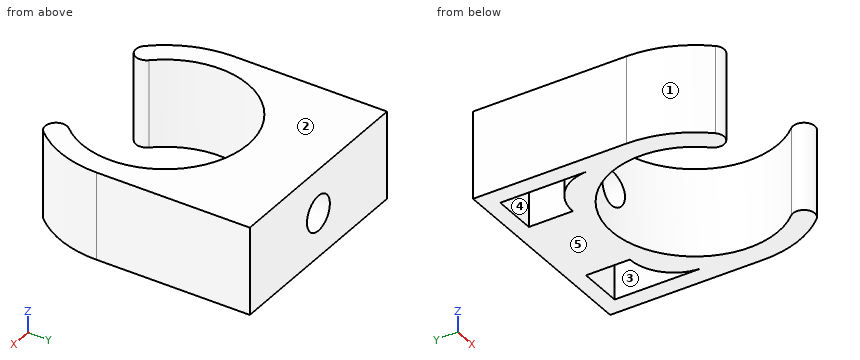
from build123d import *

# Parameters (mm, degrees)
BOSS_EXTRUDE2_DEPTH = 5
SKETCH5_R           = 2
CUT_EXTRUDE1_DEPTH  = 9
CUT_EXTRUDE2_DEPTH  = 8


with BuildPart() as part:
    # Sketch3 → Boss-Extrude2 (new, symmetric)
    with BuildSketch(Plane.XY):
        with BuildLine():
            Line((-12, -4.5), (-12, 13))
            Line((-12, 13), (12, 13))
            Line((12, 13), (12, -4.5))
            ThreePointArc((12, -4.5), (11.187544084, -8.840375258), (8.860190437, -12.593023256))
            ThreePointArc((8.860190437, -12.593023256), (7.094230677, -12.672936504), (7.014317429, -10.906976744))
            ThreePointArc((7.014317429, -10.906976744), (0, 5), (-7.014317429, -10.906976744))
            ThreePointArc((-7.014317429, -10.906976744), (-7.094230677, -12.672936504), (-8.860190437, -12.593023256))
            ThreePointArc((-8.860190437, -12.593023256), (-11.187544084, -8.840375258), (-12, -4.5))
        make_face()
    extrude(amount=BOSS_EXTRUDE2_DEPTH, both=True)

    # Sketch5 → Cut-Extrude1 (cut)
    with BuildSketch(Plane(origin=(0, 13, 0), x_dir=(1, 0, 0), z_dir=(0, 1, 0))):
        with Locations(Location((0, 0, 0), (0, 0, 270))):
            Circle(SKETCH5_R)
    extrude(amount=-CUT_EXTRUDE1_DEPTH, mode=Mode.SUBTRACT)

    # Sketch7 → Cut-Extrude2 (cut)
    with BuildSketch(Plane(origin=(0, 0, -5), x_dir=(-1, 0, 0), z_dir=(0, 0, -1))):
        with BuildLine():
            Line((10, 11.190527755), (10, 1.190527755))
            ThreePointArc((10, 1.190527755), (8.535533906, 4.726061661), (5, 6.190527755))
            Line((5, 6.190527755), (5, 11.190527755))
            Line((5, 11.190527755), (10, 11.190527755))
        make_face()
        with BuildLine():
            Line((-10, 11.190527755), (-10, 1.190527755))
            ThreePointArc((-10, 1.190527755), (-8.535533906, 4.726061661), (-5, 6.190527755))
            Line((-5, 6.190527755), (-5, 11.190527755))
            Line((-5, 11.190527755), (-10, 11.190527755))
        make_face()
    extrude(amount=-CUT_EXTRUDE2_DEPTH, mode=Mode.SUBTRACT)


solid = part.part
The model under review builds one solid part; all positions refer to its coordinate system, in mm. Face numbers are marked on the shaded views. A direction names the side the tool comes from. Coordinates: 2 decimals unless noted, no trailing zeros. Write each loop counter-clockwise with the first axis right and the second up, starting at its lowest first coordinate (ties: lowest second). Pieces come first, ordered by that corner, then holes. Notation, with made-up numbers: M 65.5,7 L 88.5,7 A27 cw 88.5,34 Z; hole C 42,72.25 d11. An arc over 180 degrees is marked long. Put each result on its own line as item: value.
1) For the marked faces 4 and 5, list the 3-axis set-ups (+Z, -Z, +X, -X, +Y, -Y) from which the entire face can be reached by the end or side of a thin tool; tool diameter is ignored.
Computed:
face 4: -Z
face 5: -Z, +X, -X, +Y, -Y
2) Add section A-A on z = 0. Give the boundary of the cut face in (x, y).
Computed:
outline: M -12,-4.5 A12 ccw -8.86,-12.59 A1.25 ccw -7.01,-10.91 A9.5 cw -2,4.79 L -2,13 L -12,13 Z; M 2,4.79 A9.5 cw 7.01,-10.91 A1.25 ccw 8.86,-12.59 A12 ccw 12,-4.5 L 12,13 L 2,13 Z; hole M -10,1.19 A5 cw -5,6.19 L -5,11.19 L -10,11.19 Z; hole M 5,6.19 A5 cw 10,1.19 L 10,11.19 L 5,11.19 Z
3) Add section D-D on y = 8. Give the boundary of the cut face in (x, z), then the cut area to 3 significant figures.
Computed:
outline: M -12,-5 L -10,-5 L -10,3 L -5,3 L -5,-5 L 5,-5 L 5,3 L 10,3 L 10,-5 L 12,-5 L 12,5 L -12,5 Z; hole C 0,0 d4
area: 147 mm2
4) Wall thickness on probe 1 along X at (y, z) = (7, 0); probe 2 along X at (y, z) = (-4.5, 0); probe 3 along Y at (x, z) = (7.75, 0.5): over which ranges is each line inside the solid? List them lowest first. Write a range as [from, to].
Computed:
probe 1: x = [-12, -10], [-5, -2], [2, 5], [10, 12]
probe 2: x = [-12, -9.5], [9.5, 12]
probe 3: y = [-12.99, -9.99], [0.99, 5.37], [11.19, 13]
5) Draft analysis for pull direction Y (two halves, no side actions). For the marked faces 1, 2 and 3, state which applies: released by +Y, released by -Y, zero draft, split by the parting line, or undercut.
Computed:
face 1: released by -Y
face 2: zero draft
face 3: undercut
6) Add section C-C on z = -2.75. Give the boundary of the cut face in (x, y).
Computed:
outline: M -12,-4.5 A12 ccw -8.86,-12.59 A1.25 ccw -7.01,-10.91 A9.5 cw long 7.01,-10.91 A1.25 ccw 8.86,-12.59 A12 ccw 12,-4.5 L 12,13 L -12,13 Z; hole M -10,1.19 A5 cw -5,6.19 L -5,11.19 L -10,11.19 Z; hole M 5,6.19 A5 cw 10,1.19 L 10,11.19 L 5,11.19 Z
7) Clearance check with flat-ended pins moving along their axes: pin 1 Ø1.5 at (x, z) = (-8.5, 0) entering from -Y; pin 2 Ø4 at (y, z) = (-7, 2) entering from -X; pin 3 Ø1.5 at (x, y) = (-7, 7.5) entering from -Z. State where each tip first meets the part, or that it passes through.
Computed:
pin 1: stops at y = -13
pin 2: stops at x = -11.99
pin 3: stops at z = 3
8) Add section B-B on y = -1.25. Give the boundary of the cut face in (x, z), then the cut area to 3 significant figures.
Computed:
outline: M -12,-5 L -8.93,-5 L -8.93,5 L -12,5 Z; M 8.93,-5 L 12,-5 L 12,5 L 8.93,5 Z
area: 61.5 mm2
